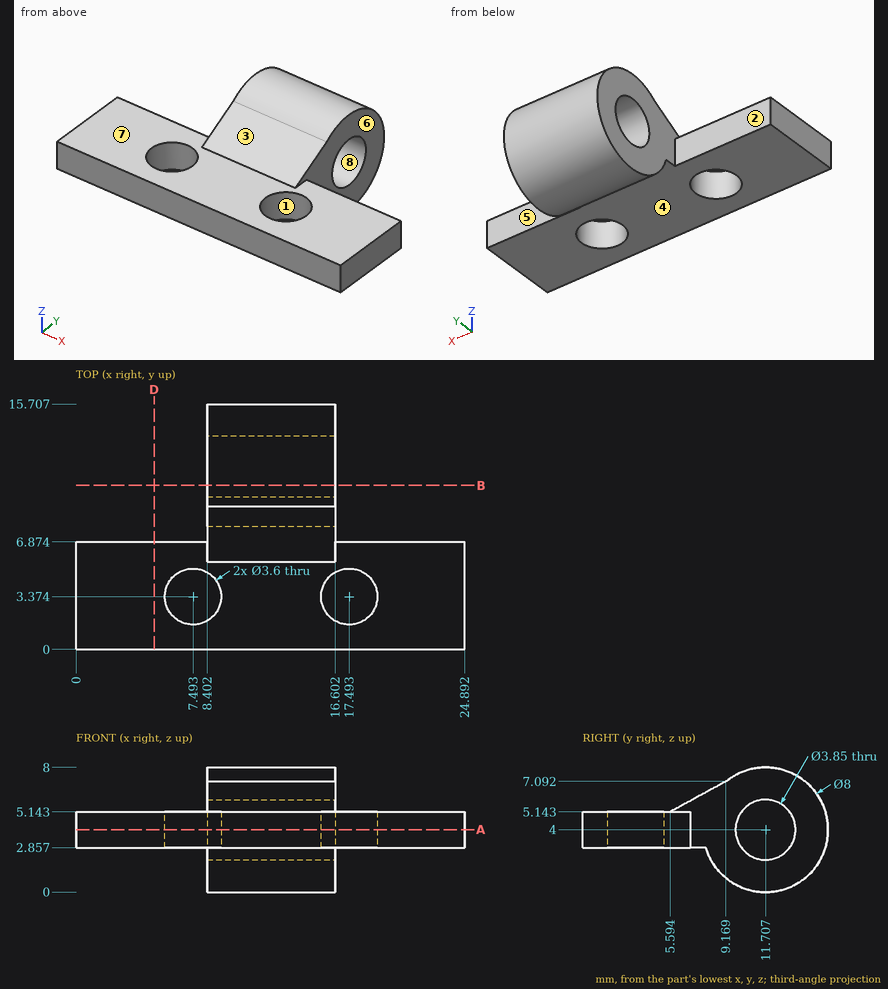
Study the drawing (mm; zero at the part's minimum x, y, z) and answer. A direction names the side the tool comes from. Coordinates: 2 decimals unless noted, no trailing zeros. Write each loop counter-clockwise with the first axis right and the second up, starting at its lowest first coordinate (ties: lowest second). Pieces come first, ordered by that corner, then holes. Notation, with made-up numbers: (65, 57) - (123, 57) arc R19 cw to (123, 86) - close; hole circle Ø5 at (-23.75, -36.5). An arc over 180 degrees is marked (long way). Answer as a JSON object with one key per item and string values.
Q1. Consider L1, parallel to Z at x = 13.75, y = 2.75; L2, parallel to Y at x = 21.75, z = 4; L3, parallel to X at y = 11.5, z = 2. Determine where each line is inside the solid, lowest interval first. Write a range as from..to.
Results list:
{"L1": "z = 2.86..5.14", "L2": "y = 0..6.87", "L3": "x = 8.4..16.6"}
Q2. Find section B-B (y = 10.5). Write down the section's boundary in (x, z).
Results list:
{"outline": "(8.4, 0.19) - (16.6, 0.19) - (16.6, 2.5) - (8.4, 2.5) - close; (8.4, 5.5) - (16.6, 5.5) - (16.6, 7.81) - (8.4, 7.81) - close"}
Q3. Find section A-A (z = 4). Write down the section's boundary in (x, y).
Results list:
{"outline": "(0, 0) - (24.89, 0) - (24.89, 6.87) - (16.6, 6.87) - (16.6, 9.78) - (8.4, 9.78) - (8.4, 6.87) - (0, 6.87) - close; (8.4, 13.63) - (16.6, 13.63) - (16.6, 15.71) - (8.4, 15.71) - close; hole circle Ø3.6 at (7.49, 3.37); hole circle Ø3.6 at (17.49, 3.37)"}
Q4. Given pin 1 Ø2.5 at (x, y) = (18, 5.5) entering from -Z; pin 2 Ø4 at (y, z) = (9.5, 6) entering from -X; pin 3 Ø1.8 at (x, z) = (20, 4.5) entering from +Y; pin 4 Ø2 at (x, z) = (12.5, 5) entering from -Y, each flat-ended and moving along its own axis, determine where each tip first touches the part or whether it passes through.
Results list:
{"pin 1": "stops at z = 2.86", "pin 2": "stops at x = 8.4", "pin 3": "stops at y = 6.87", "pin 4": "stops at y = 0"}
Q5. Find section D-D (x = 5). Write down the section's boundary in (y, z).
Results list:
{"outline": "(0, 2.86) - (6.87, 2.86) - (6.87, 5.14) - (0, 5.14) - close"}
Q6. Which of the six approach directions +Z, -Z, +X, -X, +Y, -Y give full straight-line access (tool end or side, diameter ignored) to the marked faces 1, 2, 3, 4 and 5?
Results list:
{"face 1": "+Z, -Z", "face 2": "+Z, -Z, -X, +Y", "face 3": "+Z, +X, -X, -Y", "face 4": "-Z, +X, -X, -Y", "face 5": "+Z, -Z, +X, +Y"}
Q7. For a pull along Z with two mould halves and no side action, classify the marked faces 6, 7 and 8 as pulls with the +Z half, pulls with the -Z half, needs draft (parallel to the pull), parting line crosses it, or undercut.
Results list:
{"face 6": "needs draft", "face 7": "pulls with the +Z half", "face 8": "undercut"}
